Autodesk Inventor part; units mm, degrees
ref_plane "YZ Plane" through (0, 0, 0) normal (1, 0, 0) x (0, 1, 0)
ref_plane "XZ Plane" through (0, 0, 0) normal (0, 1, 0) x (-1, 0, 0)
ref_plane "XY Plane" through (0, 0, 0) normal (0, 0, 1) x (1, 0, 0)
sketch "Boceto1" plane through (0, 0, 0) normal (0, 0, 1) x (1, 0, 0)
  circle A0 centre (0, 0) radius 25
  circle A1 centre (0, 0) radius 10
  line L0 (0, -25) -> (0, -17.5)
  circle A2 centre (0, -17.5) radius 4
  dimension "d0" = 50
  dimension "d1" = 20
  dimension "d3" = 7.5
  dimension "d4" = 8
extrude "Extrusión1" add sketch "Boceto1" along normal blind 35 contours A2
extrude "Extrusión2" add sketch "Boceto1" along normal blind 20
fillet "Empalme1" radius 1 3 edges at (-25, 0, 0) (-25, 0, 20) (-4, -17.5, 35)
sketch "Boceto3" plane through (0, 0, 20) normal (0, 0, 1) x (1, 0, 0)
  line L0 (0, 15.6) -> (-3.5, 15.6)
  line L1 (-3.5, 15.6) -> (-3.5, 5.6)
  line L2 (-3.5, 5.6) -> (3.5, 5.6)
  line L3 (3.5, 5.6) -> (3.5, 15.6)
  line L4 (3.5, 15.6) -> (0, 15.6)
  point P0 (0, 0)
  dimension "d18" = 15.6
  dimension "d19" = 3.5
  dimension "d20" = 10
  dimension "d21" = 7
extrude "Extrusión4" cut sketch "Boceto3" against normal through all
properties part number "PIEZA PARA GIRAR"
Could you check a few things on this model? Use its own coordinates, in mm. A direction names the side the tool comes from. Give positions to 0.01 mm unless a question says otherwise; leave off trailing zeros. Order: outer loops, then holes, each group sorted by start corner. A loop starts at its lowest first (then second) coordinate and runs counter-clockwise, first axis right, second up.
1. Thinking about a two-plate mould opening in Y: for faces 1 (the flat face through (3.5, 12, 10)), 2 (the cylindrical face through (-0.521, -21.466, 26.902)), 3 (the flat face through (0, -17, 35)), 4 (the flat face through (0, 15.6, 10)), which applies, +Y half, -Y half, draft (parallel to the pull), parting line (faces both ways), or undercut?
Answers below:
face 1: undercut
face 2: parting line
face 3: draft
face 4: undercut
2. Suppose I cut it at A-A (y = 0). Write out the boundary of the cut face in (x, z).
Answers below:
outline: (-25, 1) arc R1 ccw to (-24, 0) - (-10, 0) - (-10, 20) - (-24, 20) arc R1 ccw to (-25, 19) - close; (10, 0) - (24, 0) arc R1 ccw to (25, 1) - (25, 19) arc R1 ccw to (24, 20) - (10, 20) - close
3. Which directions (+Z, -Z, +X, -X, +Y, -Y) give clear straight access to the entire face, cutting with the end or side of a thin tool? Please do faces 5 (the flat face through (-0.3, -10.3, 0)), 6 (the flat face through (-3.5, 13, 10)).
Answers below:
face 5: -Z, +X, -X, +Y, -Y
face 6: +Z, -Z
4. Suppose I cut it at B-B (x = 0). Write out the boundary of the cut face in (y, z).
Answers below:
outline: (-25, 1) arc R1 ccw to (-24, 0) - (-10, 0) - (-10, 20) - (-13.5, 20) - (-13.5, 34) arc R1 ccw to (-14.5, 35) - (-20.5, 35) arc R1 ccw to (-21.5, 34) - (-21.5, 20) - (-24, 20) arc R1 ccw to (-25, 19) - close; (15.6, 0) - (24, 0) arc R1 ccw to (25, 1) - (25, 19) arc R1 ccw to (24, 20) - (15.6, 20) - close
5. Suppose I cut it at C-C (z = 14.5). Write out the boundary of the cut face in (x, y), plus the area to 3 significant figures.
Answers below:
outline: circle Ø50 at (0, 0); hole (-3.5, 9.37) arc R10 ccw (long way) to (3.5, 9.37) - (3.5, 15.6) - (-3.5, 15.6) - close
area: 1,610 mm2
6. For pin 1 (1.5 mm diameter, centred on x = -14, z = 18, fed in from +Y); pin 2 (3 mm diameter, centred on y = 12, z = 9.5, fed in from +X); pin 3 (6 mm diameter, centred on x = 12, y = -1.5, fed in from +Z); pin 4 (18 mm diameter, centred on x = 0, y = 0, fed in from -Z), each with a flat end and sliding along its axis, tell me the tip position at first contact or that it passes through.
Answers below:
pin 1: stops at y = 21.2
pin 2: stops at x = 22.69
pin 3: stops at z = 20
pin 4: passes through
7. I need wall thicknesses on L1, parallel to X at y = 15, z = 16.5; L2, parallel to Y at x = -1.5, z = 10; L3, parallel to X at y = -5, z = 17.5. Which ranges of each line are inside material? Lowest first, please.
Answers below:
L1: x = -20 to -3.5, 3.5 to 20
L2: y = -24.95 to -9.89, 15.6 to 24.95
L3: x = -24.49 to -8.66, 8.66 to 24.49
8. Suppose I cut it at D-D (z = 25.5). Write out the boundary of the cut face in (x, y).
Answers below:
outline: circle Ø8 at (0, -17.5)
